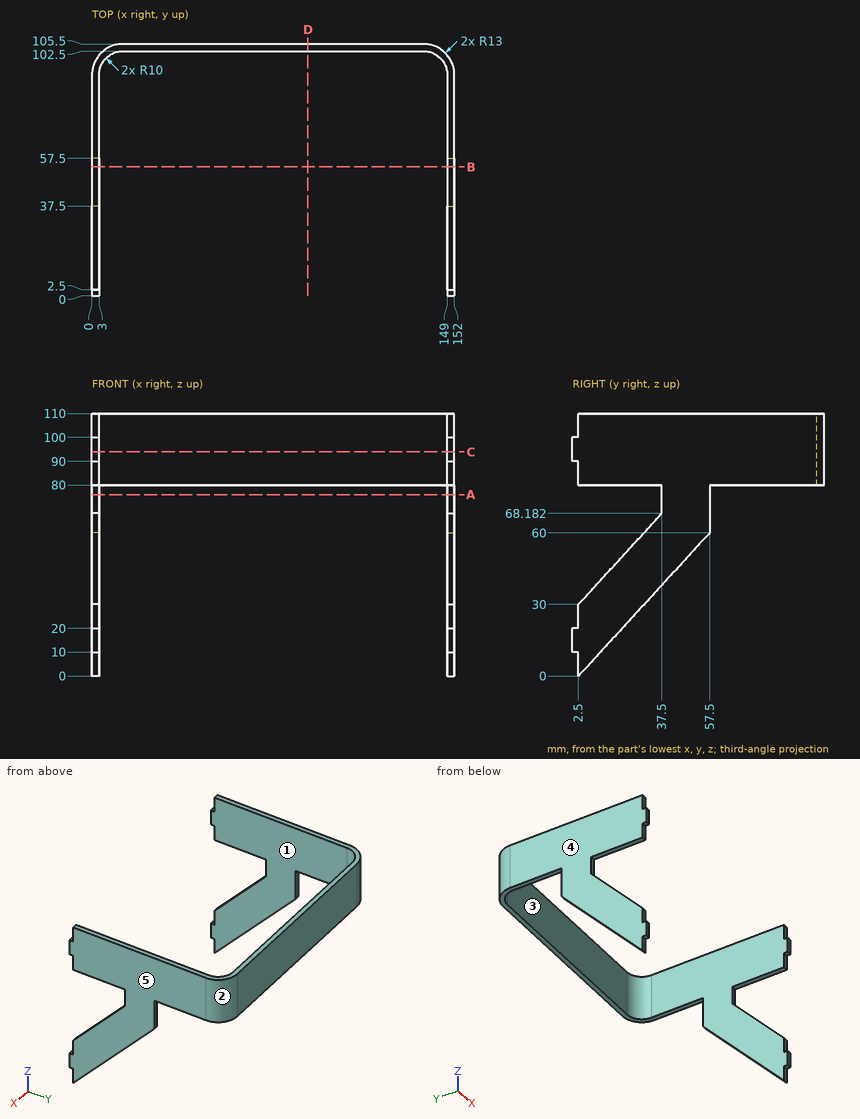
Input: dimensioned drawing with shaded views. Units: mm. Origin: part minimum x, y, z. A direction names the side the tool comes from. Coordinates: 2 decimals unless noted, no trailing zeros. Order: outer loops, then holes, each group sorted by start corner. A loop starts at its lowest first (then second) coordinate and runs counter-clockwise, first axis right, second up. Notation, with made-up numbers: (1.5, -31) - (41.5, -31) arc R8 cw to (41.5, -17) - close; hole circle Ø1 at (71.25, 15.5). An arc over 180 degrees is marked (long way). One line per item, written item: value.
1) Cut plane C-C on z = 94. Output: boundary loops of the cut face in (x, y).
Computed values:
outline: (0, 0) - (3, 0) - (3, 92.5) arc R10 cw to (13, 102.5) - (139, 102.5) arc R10 cw to (149, 92.5) - (149, 0) - (152, 0) - (152, 92.5) arc R13 ccw to (139, 105.5) - (13, 105.5) arc R13 ccw to (0, 92.5) - close
2) Ray query, line 1 (X direction, y = 28, z = 87); line 2 (Y direction, x = 98, z = 101). Return the intervals inside material, ascending. Write a range as [from, to].
Computed values:
line 1: x = [0, 3], [149, 152]
line 2: y = [102.5, 105.5]
3) Cut plane D-D on x = 90.5. Output: boundary loops of the cut face in (y, z), plus the area to 3 significant figures.
Computed values:
outline: (102.5, 80) - (105.5, 80) - (105.5, 110) - (102.5, 110) - close
area: 90.0 mm^2
4) Mould query, pull axis X, two halves, no side actions, for the marked faces 3, 4 and 5. Classes: released by +X, released by -X, zero draft, split by the parting line, or undercut.
Computed values:
face 3: undercut
face 4: released by -X
face 5: released by +X
5) Cut plane A-A on z = 76. Output: boundary loops of the cut face in (x, y), plus the area to 3 significant figures.
Computed values:
outline: (0, 37.5) - (3, 37.5) - (3, 57.5) - (0, 57.5) - close; (149, 37.5) - (152, 37.5) - (152, 57.5) - (149, 57.5) - close
area: 120 mm^2
6) Reachability of the marked faces 1 and 2 from +Z, -Z, +X, -X, +Y, -Y: full face, straight path, thin tool, end or side. Return the list, or none.
Computed values:
face 1: +Z, -Z, -Y
face 2: +Z, -Z, +X, +Y
7) Contact query for flat-ended pins moving along their axis: pin 1 (3.5 mm diameter, centred on x = 1.5, z = 87, fed in from -Y); pin 2 (3 mm diameter, centred on y = 30, z = 46, fed in from -X); pin 3 (2.5 mm diameter, centred on x = 150.5, z = 65, fed in from +Y); pin 4 (2 mm diameter, centred on x = 1, y = 1, fed in from -Z). Output: stop coordinate, or through.
Computed values:
pin 1: stops at y = 2.5
pin 2: stops at x = 0
pin 3: stops at y = 57.5
pin 4: stops at z = 10
8) Cut plane B-B on y = 54. Output: boundary loops of the cut face in (x, z), plus the area to 3 significant figures.
Computed values:
outline: (0, 56.18) - (3, 56.18) - (3, 110) - (0, 110) - close; (149, 56.18) - (152, 56.18) - (152, 110) - (149, 110) - close
area: 323 mm^2
